from build123d import *

# Parameters (mm, degrees)
SKETCH_1_W          = 20
SKETCH_1_H          = 20
SKETCH_1_W_2        = 18
SKETCH_1_H_2        = 18
EXTRUDE_2_DEPTH     = 277
SKETCH_2_R          = 2.65
SKETCH_2_R_2        = 1.1
CUT_EXTRUDE_1_DEPTH = 20
SKETCH_5_R          = 2.65
CUT_EXTRUDE_2_DEPTH = 20
SKETCH_6_R          = 6
CUT_EXTRUDE_3_DEPTH = 10


with BuildPart() as part:
    # 草图1 → 凸台-拉伸2 (new body)
    with BuildSketch(Plane.XY):
        with Locations((10, -10)):
            Rectangle(SKETCH_1_W, SKETCH_1_H)
        with Locations((10, -10)):
            Rectangle(SKETCH_1_W_2, SKETCH_1_H_2, mode=Mode.SUBTRACT)
    extrude(amount=EXTRUDE_2_DEPTH)

    # 草图2 → 切除-拉伸1 (cut)
    with BuildSketch(Plane(origin=(0, -20, 0), x_dir=(-1, 0, 0), z_dir=(0, -1, 0))):
        with Locations(Location((-10, -9, 0), (0, 0, 90))):
            Circle(SKETCH_2_R)
        with Locations(Location((-10, -24, 0), (0, 0, 90))):
            Circle(SKETCH_2_R)
        with Locations(Location((-10, -39, 0), (0, 0, 90))):
            Circle(SKETCH_2_R)
        with Locations(Location((-10, -54, 0), (0, 0, 90))):
            Circle(SKETCH_2_R)
        with Locations(Location((-10, -69, 0), (0, 0, 90))):
            Circle(SKETCH_2_R)
        with Locations(Location((-10, -99, 0), (0, 0, 90))):
            Circle(SKETCH_2_R_2)
        with Locations(Location((-10, -129, 0), (0, 0, 90))):
            Circle(SKETCH_2_R_2)
        with Locations(Location((-10, -144, 0), (0, 0, 90))):
            Circle(SKETCH_2_R_2)
        with Locations(Location((-10, -174, 0), (0, 0, 90))):
            Circle(SKETCH_2_R_2)
        with Locations(Location((-10, -189, 0), (0, 0, 90))):
            Circle(SKETCH_2_R_2)
        with Locations(Location((-10, -219, 0), (0, 0, 90))):
            Circle(SKETCH_2_R_2)
        with Locations(Location((-10, -234, 0), (0, 0, 90))):
            Circle(SKETCH_2_R_2)
        with Locations(Location((-10, -249, 0), (0, 0, 90))):
            Circle(SKETCH_2_R_2)
        with Locations(Location((-10, -84, 0), (0, 0, 90))):
            Circle(SKETCH_2_R_2)
        with Locations(Location((-10, -259, 0), (0, 0, 90))):
            Circle(SKETCH_2_R_2)
        with Locations(Location((-10, -274, 0), (0, 0, 90))):
            Circle(SKETCH_2_R_2)
    extrude(amount=-CUT_EXTRUDE_1_DEPTH, mode=Mode.SUBTRACT)

    # 草图5 → 切除-拉伸2 (cut)
    with BuildSketch(Plane.ZY):
        with Locations(Location((9, -10, 0), (0, 0, 270))):
            Circle(SKETCH_5_R)
        with Locations(Location((24, -10, 0), (0, 0, 270))):
            Circle(SKETCH_5_R)
        with Locations(Location((39, -10, 0), (0, 0, 270))):
            Circle(SKETCH_5_R)
        with Locations(Location((54, -10, 0), (0, 0, 270))):
            Circle(SKETCH_5_R)
    extrude(amount=-CUT_EXTRUDE_2_DEPTH, mode=Mode.SUBTRACT)

    # 草图6 → 切除-拉伸3 (cut)
    with BuildSketch(Plane(origin=(0, -20, 0), x_dir=(-1, 0, 0), z_dir=(0, -1, 0))):
        with Locations(Location((-10, -39, 0), (0, 0, 90))):
            Circle(SKETCH_6_R)
        with Locations(Location((-10, -54, 0), (0, 0, 90))):
            Circle(SKETCH_6_R)
        with Locations(Location((-10, -69, 0), (0, 0, 90))):
            Circle(SKETCH_6_R)
    extrude(amount=-CUT_EXTRUDE_3_DEPTH, mode=Mode.SUBTRACT)


solid = part.part
Model file for the job. Use its own axes, mm. A direction names the side the tool comes from. Coordinates: 2 decimals unless noted, no trailing zeros. Write each loop counter-clockwise with the first axis right and the second up, starting at its lowest first coordinate (ties: lowest second). Pieces come first, ordered by that corner, then holes. Notation, with made-up numbers: (0.25, -35) -> (27.25, -35) arc R27 cw to (27.25, -19) -> close; hole circle Ø11 at (45, 69.25). An arc over 180 degrees is marked (long way). One line per item, written item: value. Start each with the question number.
1) Probe probe 1 along X at (y, z) = (-11, 33.5); probe 2 along X at (y, z) = (-19.55, 69); probe 3 along Z at (x, y) = (19.55, -10). List the from-to ranges inside material, lowest first.
2) Which spindle directions (+Z, -Z, +X, -X, +Y, -Y) get a long thin tool onto all of the face, cutting with end or side? Do faces 4 (the face through (1, -10, 137)), 5 (the face through (6.35, -19.51, 43.76)), 6 (the face through (0.49, -9.66, 56.63)). Say none if no direction does.
3) Slice it at A-A on z = 69. Write the cut outline in (x, y).
4) Slice it at B-B on y = -4.25. Write the cut outline in (x, z), then the cut area to 3 significant figures.
5) Pull direction Z, two halves, no side cores. Call faces 1 (the face through (0, -10, 137)), 2 (the face through (6.35, -19.51, 58.76)), 3 (the face through (9.2, -19.6, 0)): +Z half, -Z half, draft (parallel to the pull), parting line (faces both ways), or undercut.
6) Flat gauge pins, fed straight in: pin 1 Ø7 at (x, z) = (10, 54) entering from +Y; pin 2 Ø7 at (x, z) = (10, 54) entering from -Y. Where does each tip first touch, or does it go through?
7) Slice it at D-D on z = 24. Write the cut outline in (x, y), then the cut area to 3 significant figures.
8) Slice it at C-C on z = 162.5. Write the cut outline in (x, y).
Answers follow:
1. probe 1: 0 to 1, 19 to 20
1. probe 2: 0 to 4, 16 to 20
1. probe 3: 0 to 6.35, 11.65 to 21.35, 26.65 to 36.35, 41.65 to 51.35, 56.65 to 277
2. face 4: +Z, -Z
2. face 5: -Y
2. face 6: +X, -X
3. outline: (0, -20) -> (4, -20) -> (4, -19) -> (1, -19) -> (1, -1) -> (7.35, -1) -> (7.35, 0) -> (0, 0) -> close; (12.65, -1) -> (19, -1) -> (19, -19) -> (16, -19) -> (16, -20) -> (20, -20) -> (20, 0) -> (12.65, 0) -> close
4. outline: (0, 0) -> (1, 0) -> (1, 277) -> (0, 277) -> close; (19, 0) -> (20, 0) -> (20, 277) -> (19, 277) -> close
4. area: 554 mm2
5. face 1: draft
5. face 2: undercut
5. face 3: -Z half
6. pin 1: y = 0
6. pin 2: y = -1
7. outline: (0, -20) -> (7.35, -20) -> (7.35, -19) -> (1, -19) -> (1, -12.65) -> (0, -12.65) -> close; (0, -7.35) -> (1, -7.35) -> (1, -1) -> (7.35, -1) -> (7.35, 0) -> (0, 0) -> close; (12.65, -20) -> (20, -20) -> (20, -12.65) -> (19, -12.65) -> (19, -19) -> (12.65, -19) -> close; (12.65, -1) -> (19, -1) -> (19, -7.35) -> (20, -7.35) -> (20, 0) -> (12.65, 0) -> close
7. area: 54.8 mm2
8. outline: (0, -20) -> (20, -20) -> (20, 0) -> (0, 0) -> close; hole (1, -19) -> (19, -19) -> (19, -1) -> (1, -1) -> close
